Could you check a few things on this model? Use its own coordinates, in mm. A direction names the side the tool comes from. Give positions to 0.01 mm unless a question says otherwise; leave off trailing zeros. Order: outer loops, then holes, each group sorted by start corner. A loop starts at its lowest first (then second) coordinate and runs counter-clockwise, first axis right, second up. Notation, with made-up numbers: M 88.5,81.25 L 108.5,81.25 A16 cw 108.5,105.25 Z; hole C 0.25,89 d9. An arc over 180 degrees is marked long. Return JSON: item names as keys, results as strings. Group by question number.
```python
from build123d import *

# Parameters (mm, degrees)
F1_DEPTH = 19.05
F2_R     = 50.8
F3_W     = 88.9
F3_H     = 38.1
F4_DEPTH = 38.1
F5_W     = 38.1
F5_H     = 76.2
F6_DEPTH = 38.101


with BuildPart() as f1:
    # F0 (on Front) → F1 (new body, symmetric)
    with BuildSketch(Plane.XZ):
        Polygon((-76.2, 0), (-19.05, 0), (19.05, 0), (76.2, 0), (330.2, -433.689813), (381, -433.689813), (168.919206, 76.2), (381, 290.210187), (292.1, 290.210187), (65.278791, 152.4), (0, 152.4), (-65.278791, 152.4), (-292.1, 290.210187), (-381, 290.210187), (-168.919206, 76.2), (-381, -433.689813), (-330.2, -433.689813), align=None)
    extrude(amount=F1_DEPTH, both=True)

    # F2
    f2_edges = [f1.edges().sort_by_distance(p)[0] for p in [
        (168.919206, 0, 76.2),
        (-65.278791, 0, 152.4),
        (65.278791, 0, 152.4),
        (-168.919206, 0, 76.2),
        (-76.2, 0, 0),
        (76.2, 0, 0),
    ]]
    fillet(f2_edges, radius=F2_R)

    # F3 (on face) → F4 (join)
    with BuildSketch(Plane.XY.offset(290.210187)):
        with Locations((-336.55, 0)):
            Rectangle(F3_W, F3_H)
        with Locations((336.55, 0)):
            Rectangle(F3_W, F3_H)
    extrude(amount=F4_DEPTH)

    # F5 (on face) → F6 (cut, through all)
    with BuildSketch(Plane.XZ.offset(19.05)):
        with Locations((0, 114.3)):
            Rectangle(F5_W, F5_H)
    extrude(amount=-F6_DEPTH, mode=Mode.SUBTRACT)


solid = f1.part
```
1. If we mould it in two halves opening along Z, with no side actions, what happens to faces 1 (the cylindrical face through (-72.022, 0.267, -6.544)), 2 (the flat face through (-292.1, 0, 309)), 3 (the flat face through (35, 0, 152.4)), 4 (the cylindrical face through (179.045, -0.267, 74.643))? For each: pulls with the +Z half, pulls with the -Z half, needs draft (parallel to the pull), parting line crosses it, or undercut.
2. Imagine slicing it at C-C, the plane y = -6. Please give me the cut outline in (x, z), plus the area to 3 significant figures.
3. For pin 1 (4 mm diameter, centred on y = -11.5, z = -29.5, fed in from -X); pin 2 (10 mm diameter, centred on x = 237, y = 15, fed in from -Z); pin 3 (12 mm diameter, centred on x = -258.5, y = -14, fed in from -Z), each with a flat end and sliding along its axis, tell me the tip position at first contact or that it passes through.
4. Which directions (+Z, -Z, +X, -X, +Y, -Y) give clear straight access to the entire face, cutting with the end or side of a thin tool? Please do faces 5 (the flat face through (-19.05, 0, 114)), 6 (the flat face through (-280.06, -0.27, -191.01)), 7 (the flat face through (282.85, -0.27, -197.71)), 8 (the flat face through (-1, 0, 0)).
5. Imagine slicing it at A-A, the plane z = -192.5. Please give me the cut outline in (x, y).
6. Imagine slicing it at B-B, the plane x = -260. Please give me the cut outline in (y, z).
7. I need wall thicknesses on L1, parallel to Z at x = -267, y = 3; L2, parallel to X at y = -5, z = 265.5; L3, parallel to X at y = 16, z = -155.5. Which ranges of each line are inside material? Lowest first, please. Write a range as from..to.
8. Imagine slicing it at D-D, the plane x = 6.5. Please give me the cut outline in (y, z), plus the area to 3 significant figures.
Values:
{
 "1": {"face 1": "pulls with the -Z half", "face 2": "needs draft", "face 3": "pulls with the +Z half", "face 4": "undercut"},
 "2": {"outline": "M -381,-433.69 L -330.2,-433.69 L -90.92,-25.13 A50.8 cw -47.08,0 L 47.08,0 A50.8 cw 90.92,-25.13 L 330.2,-433.69 L 381,-433.69 L 181.91,44.96 A50.8 cw 192.73,100.23 L 381,290.21 L 381,328.31 L 292.1,328.31 L 292.1,290.21 L 77.43,159.79 A50.8 cw 51.06,152.4 L 19.05,152.4 L 19.05,76.2 L -19.05,76.2 L -19.05,152.4 L -51.06,152.4 A50.8 cw -77.43,159.79 L -292.1,290.21 L -292.1,328.31 L -381,328.31 L -381,290.21 L -192.73,100.23 A50.8 cw -181.91,44.96 Z", "area": "177,000 mm²"},
 "3": {"pin 1": "stops at x = -213.72", "pin 2": "stops at z = -283.09", "pin 3": "stops at z = -321.51"},
 "4": {"face 5": "+Z, +Y, -Y", "face 6": "-X, +Y, -Y", "face 7": "+X, +Y, -Y", "face 8": "-Z, +Y, -Y"},
 "5": {"outline": "M -280.68,-19.05 L -188.94,-19.05 L -188.94,19.05 L -280.68,19.05 Z; M 188.94,-19.05 L 280.68,-19.05 L 280.68,19.05 L 188.94,19.05 Z"},
 "6": {"outline": "M -19.05,-313.83 L 19.05,-313.83 L 19.05,-142.78 L -19.05,-142.78 Z; M -19.05,168.11 L 19.05,168.11 L 19.05,270.71 L -19.05,270.71 Z"},
 "7": {"L1": "z = -325.78..-159.61, 175.17..274.96", "L2": "x = -356.51..-251.43, 251.43..356.51", "L3": "x = -265.29..-167.27, 167.27..265.29"},
 "8": {"outline": "M -19.05,0 L 19.05,0 L 19.05,76.2 L -19.05,76.2 Z", "area": "2,900 mm²"}
}
